Design review of the part built by this model. Coordinates are the model's own, in mm. A direction names the side the tool comes from. Give positions to 0.01 mm unless a question says otherwise; leave off trailing zeros. Write each loop counter-clockwise with the first axis right and the second up, starting at its lowest first coordinate (ties: lowest second). Pieces come first, ordered by that corner, then holes.
```python
from build123d import *

# Parameters (mm, degrees)
F0_W     = 18
F0_H     = 52
F0_W_2   = 8
F0_H_2   = 40
F1_DEPTH = 3
F2_W     = 2
F2_H     = 8
F3_DEPTH = 15


with BuildPart() as f1:
    # F0 (on Front) → F1 (new body)
    with BuildSketch(Plane.XZ):
        Rectangle(F0_W, F0_H)
        Rectangle(F0_W_2, F0_H_2, mode=Mode.SUBTRACT)
    extrude(amount=F1_DEPTH)

    # F2 (on face) → F3 (join)
    with BuildSketch(Plane(origin=(0, 0, 0), x_dir=(-1, 0, 0), z_dir=(0, 1, 0))):
        with Locations((-8, 22)):
            Rectangle(F2_W, F2_H)
        with Locations((8, 22)):
            Rectangle(F2_W, F2_H)
        with Locations((8, -22)):
            Rectangle(F2_W, F2_H)
        with Locations((-8, -22)):
            Rectangle(F2_W, F2_H)
    extrude(amount=F3_DEPTH)


solid = f1.part
```
(1) Clearance check with flat-ended pins moving along their axes: P1, Ø5.5, axis at x = 0, z = -8, coming from the +Y side; P2, Ø8, axis at x = -2, z = 19.5, coming from the +Y side; P3, Ø4, axis at y = 1.5, z = 5.5, coming from the +X side. State where each tip first meets the part, or that it passes through.
Resolved:
P1: passes through
P2: stops at y = 0
P3: stops at x = 9
(2) To check wall thickness, follow L1, parallel to X at y = 6, z = 21; L2, parallel to Z at x = 7.5, y = 5.5; L3, parallel to Y at x = 8, z = 13. State the ranges of each line that lie inside material, in increasing order.
Resolved:
L1: x = -9 to -7, 7 to 9
L2: z = -26 to -18, 18 to 26
L3: y = -3 to 0
(3) Consider section D-D, the plane x = 5. Give the boundary of the cut face in (y, z).
Resolved:
outline: (-3, -26) - (0, -26) - (0, 26) - (-3, 26) - close
(4) Consider section A-A, the plane y = 4.75. Give the boundary of the cut face in (x, z), then the cut area to 3 significant figures.
Resolved:
outline: (-9, -26) - (-7, -26) - (-7, -18) - (-9, -18) - close; (-9, 18) - (-7, 18) - (-7, 26) - (-9, 26) - close; (7, -26) - (9, -26) - (9, -18) - (7, -18) - close; (7, 18) - (9, 18) - (9, 26) - (7, 26) - close
area: 64.0 mm2
(5) Mouldability with a two-part tool opening along Z and no side actions: class faces 1 (the face through (8, 7, 18)), 2 (the face through (1, -1, -26)), 3 (the face through (-9, -1, 0)) as pulls with the +Z half, pulls with the -Z half, needs draft (parallel to the pull), parting line crosses it, or undercut.
Resolved:
face 1: undercut
face 2: pulls with the -Z half
face 3: needs draft
(6) Tool access review of faces 4 (the face through (0, -1, -20)), 5 (the face through (-7, 7, -22)), 6 (the face through (9, -2, 0)), 7 (the face through (8, 7, -18)): name each direction out of +Z, -Z, +X, -X, +Y, -Y from which nothing blocks a thin tool from reaching the whole face with its end or side.
Resolved:
face 4: +Y, -Y
face 5: +Z, -Z, +Y
face 6: +Z, -Z, +X, +Y, -Y
face 7: +X, -X, +Y
(7) Consider section C-C, the plane x = -0.25. Give the boundary of the cut face in (y, z).
Resolved:
outline: (-3, -26) - (0, -26) - (0, -20) - (-3, -20) - close; (-3, 20) - (0, 20) - (0, 26) - (-3, 26) - close
(8) Consider section B-B, the plane z = 7. Give the boundary of the cut face in (x, y), then the cut area to 3 significant figures.
Resolved:
outline: (-9, -3) - (-4, -3) - (-4, 0) - (-9, 0) - close; (4, -3) - (9, -3) - (9, 0) - (4, 0) - close
area: 30.0 mm2
